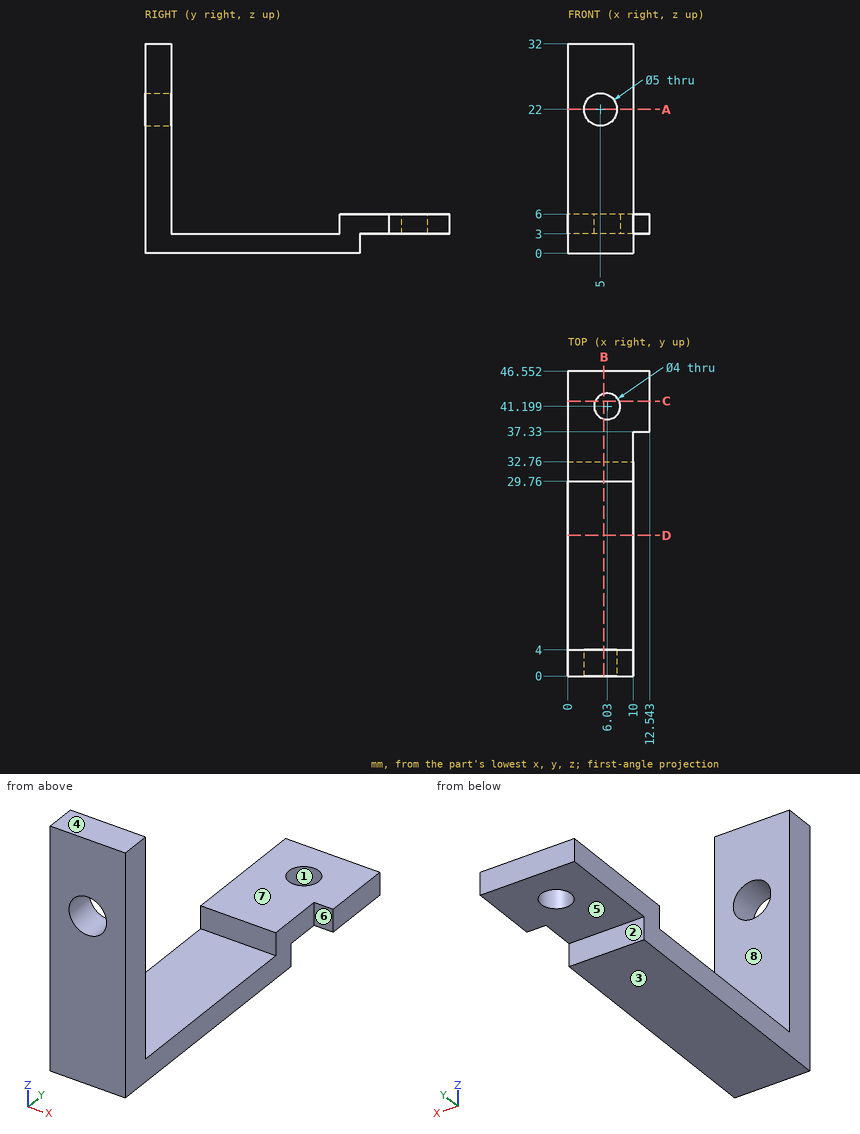
Answer from the drawing. Dimensions are ordinates in mm from the lowest x, y and z of the part. A direction names the side the tool comes from. Round coordinates to 2 decimals unless told otherwise and drop trailing zeros. Order: outer loops, then holes, each group sorted by start corner. A loop starts at its lowest first (then second) coordinate and runs counter-clockwise, first axis right, second up. Notation, with made-up numbers: (5.5, 32.25) - (45.5, 32.25) arc R16 ccw to (45.5, 56.25) - close; hole circle Ø9 at (27.25, 85). An arc over 180 degrees is marked (long way). Put each result on its own line as item: value. Start each with the question number.
(1) Given P1, Ø1.3, axis at x = 11, z = 4.5, coming from the -Y side; P2, Ø6.5, axis at x = 9, y = 39, coming from the +Z side; P3, Ø6, axis at x = 5, z = 22, coming from the +Y side, each flat-ended and moving along its own axis, determine where each tip first touches the part or whether it passes through.
(2) Find section A-A (z = 22). Give the vertices of the cut face in (x, y).
(3) Find section D-D (y = 21.5). Give the vertices of the cut face in (x, z), plus the area to 3 significant figures.
(4) Find section C-C (y = 42). Give the vertices of the cut face in (x, z).
(5) Find section B-B (x = 5.5). Give the vertices of the cut face in (y, z).
(6) For the marked faces 4, 5, 6, 7 and 8, determine the directions among +Z, -Z, +X, -X, +Y, -Y from which every point of the face is accessible in a straight line to the end or side of a thin tool.
(7) Straight lines are drawn through the part: probe 1 along Y at (x, z) = (7, 4.5); probe 2 along Z at (x, y) = (5, 1.1); probe 3 along Y at (x, z) = (5.5, 4). For each, find the intervals that lie inside material, in ascending order. Write a range as from..to.
(8) Determine the mould class of the marked faces 1, 2 and 3 for opening direction Y: released by +Y, released by -Y, zero draft, split by the parting line, or undercut.
Reply:
1. P1: y = 37.33
1. P2: z = 6
1. P3: y = 4
2. outline: (0, 0) - (2.5, 0) - (2.5, 4) - (0, 4) - close; (7.5, 0) - (10, 0) - (10, 4) - (7.5, 4) - close
3. outline: (0, 0) - (10, 0) - (10, 3) - (0, 3) - close
3. area: 30.0 mm^2
4. outline: (0, 3) - (4.2, 3) - (4.2, 6) - (0, 6) - close; (7.86, 3) - (12.54, 3) - (12.54, 6) - (7.86, 6) - close
5. outline: (0, 0) - (32.76, 0) - (32.76, 3) - (39.27, 3) - (39.27, 6) - (29.76, 6) - (29.76, 3) - (4, 3) - (4, 19.55) - (0, 19.55) - close; (0, 24.45) - (4, 24.45) - (4, 32) - (0, 32) - close; (43.13, 3) - (46.55, 3) - (46.55, 6) - (43.13, 6) - close
6. face 4: +Z, +X, -X, +Y, -Y
6. face 5: -Z, +X, -X, +Y
6. face 6: +Z, -Z, +X, -Y
6. face 7: +Z, +X, -X, +Y
6. face 8: +Z, +X, -X
7. probe 1: 0..4, 29.76..39.45, 42.95..46.55
7. probe 2: 0..19.5, 24.5..32
7. probe 3: 0..4, 29.76..39.27, 43.13..46.55
8. face 1: undercut
8. face 2: released by +Y
8. face 3: zero draft
